```python
from build123d import *

# Parameters (mm, degrees)
FILLET1_R          = 2
FILLET2_R          = 2
REVOLVE3_ANGLE     = 34.5
CUT_EXTRUDE1_START = 17.048322615
CUT_EXTRUDE1_DEPTH = 62.951677385
CUT_EXTRUDE2_REACH = 148.807
SKETCH6_W          = 2.656451676
SKETCH6_H          = 26.566734065
SKETCH6_W_2        = 2.656451675
CUT_EXTRUDE4_DEPTH = 3.1


with BuildPart() as part:
    # Sketch3 → Revolve2 (revolve)
    with BuildSketch(Plane(origin=(0, 0, 0), x_dir=(0, 0, -1), z_dir=(1, 0, 0))):
        with BuildLine():
            Line((0, 0), (36, 0))
            Line((36, 0), (36, 76.3))
            ThreePointArc((36, 76.3), (38.3, 78.6), (36, 80.9))
            Line((36, 80.9), (34.6, 80.9))
            Line((34.6, 80.9), (34.6, 76.3))
            Line((34.6, 76.3), (34.6, 1.4))
            Line((34.6, 1.4), (0, 1.4))
            Line((0, 1.4), (0, 0))
        make_face()
    revolve(axis=Axis((0, 0, 0), (0, 1, 0)))

    # Fillet1
    # the kernel refuses this fillet: 2 mm, written as the material it takes off along each edge
    with BuildSketch(Plane(origin=(0, 80.9, 0), x_dir=(0, 0, -1), z_dir=(1, 0, 0))) as fillet1_piece_1:
        with BuildLine():
            CenterArc((36.6, -1.907878403), FILLET1_R, 107.457603124, 72.542396876)
            Line((34.6, -1.907878403), (34.56, -1.907878403))
            Line((34.56, -1.907878403), (34.56, 0))
            Line((34.56, 0), (34.6, 0.04))
            ThreePointArc((34.6, 0.04), (35.3, 0.04), (35.988, 0.038157568))
            Line((35.988, 0.038157568), (36, 0))
        make_face()
    revolve(axis=Axis((0, 80.9, 0), (0, 1, 0)), mode=Mode.SUBTRACT)

    # Fillet2
    fillet2_edges = [part.edges().sort_by_distance(p)[0] for p in [
        (0, 0, 36),
    ]]
    fillet(fillet2_edges, radius=FILLET2_R)

    # Sketch4 → Revolve3 (revolve)
    with BuildSketch(Plane(origin=(0, 0, 0), x_dir=(0, 0, -1), z_dir=(1, 0, 0))):
        with BuildLine():
            Line((66.418368133, 32.345231294), (37.015359732, 17.048322615))
            Line((37.015359732, 17.048322615), (36, 9))
            Line((36, 9), (36, 19))
            Line((36, 19), (65.403008401, 34.296908679))
            ThreePointArc((65.403008401, 34.296908679), (68.549568046, 37.242877581), (69.710791194, 41.393917351))
            Line((69.710791194, 41.393917351), (69.710791194, 61.739552218))
            ThreePointArc((69.710791194, 61.739552218), (67.034063035, 68.549081537), (60.436853284, 71.71315908))
            Line((60.436853284, 71.71315908), (36, 73.492121597))
            Line((36, 73.492121597), (36, 75.686315107))
            Line((36, 75.686315107), (36.15973366, 75.686315107))
            Line((36.15973366, 75.686315107), (60.596586944, 73.90735259))
            ThreePointArc((60.596586944, 73.90735259), (68.64518284, 70.047177987), (71.910791194, 61.739552218))
            Line((71.910791194, 61.739552218), (71.910791194, 41.393917351))
            ThreePointArc((71.910791194, 41.393917351), (70.43023168, 36.101341644), (66.418368133, 32.345231294))
        make_face()
    revolve(axis=Axis((0, 0, 0), (0, 1, 0)), revolution_arc=REVOLVE3_ANGLE)

    # Cut-Extrude1: read off the stored shape, not the designer's step
    # Cut-Extrude1 outline → Cut-Extrude1 (cut)
    with BuildSketch(Plane(origin=(0, 0, 0), x_dir=(1, 0, 0), z_dir=(0, 1, 0)).offset(CUT_EXTRUDE1_START)):
        with BuildLine():
            Line((-22.108668816, 32.168312739), (-32.047363038, 63.91139403))
            Line((-32.047363038, 63.91139403), (-34.272292741, 63.218445413))
            ThreePointArc((-34.272292741, 63.218445413), (-37.553605301, 61.326084329), (-40.730720635, 59.263566268))
            Line((-40.730720635, 59.263566268), (-22.108668816, 32.168312739))
        make_face()
        with BuildLine():
            Line((0, 38.304663112), (0, 71.910791194))
            ThreePointArc((0, 71.910791194), (-3.848061143, 71.807759438), (-7.685095499, 71.498959414))
            Line((-7.685095499, 71.498959414), (-10.221387179, 70.709037913))
            Line((-10.221387179, 70.709037913), (-0.068922433, 38.283197398))
            Line((-0.068922433, 38.283197398), (0, 38.304663112))
        make_face()
    extrude(amount=CUT_EXTRUDE1_DEPTH, mode=Mode.SUBTRACT)

    # Cut-Extrude2: up to this plane
    cut_extrude2_end = Plane(origin=(-22.697932128, 11.704801269, -66.823250171), z_dir=(0.2973592990807489, 0, 0.9547656504348101))
    # Sketch6 → Cut-Extrude2 (cut, up to the surface)
    with BuildSketch(Plane(origin=(-21.486572607, 0, -68.625717394), x_dir=(-0.9543173737069837, 0, 0.2987948296758254), z_dir=(-0.2987948296758254, 0, -0.9543173737069837)), mode=Mode.PRIVATE) as cut_extrude2_sk1:
        with Locations((-12.701273409, 51.798619412)):
            Rectangle(SKETCH6_W, SKETCH6_H)
    cut_extrude2_tool1 = split(extrude(cut_extrude2_sk1.sketch, amount=-CUT_EXTRUDE2_REACH, mode=Mode.PRIVATE), bisect_by=cut_extrude2_end, keep=Keep.BOTH, mode=Mode.PRIVATE)
    add(cut_extrude2_tool1.solids().sort_by_distance((-9.365527, 51.798619, -72.420792))[0], mode=Mode.SUBTRACT)
    # Sketch6 → Cut-Extrude2 (cut, up to the surface)
    with BuildSketch(Plane(origin=(-21.486572607, 0, -68.625717394), x_dir=(-0.9543173737069837, 0, 0.2987948296758254), z_dir=(-0.2987948296758254, 0, -0.9543173737069837)), mode=Mode.PRIVATE) as cut_extrude2_sk2:
        with Locations((12.815187073, 51.798619412)):
            Rectangle(SKETCH6_W_2, SKETCH6_H)
    cut_extrude2_tool2 = split(extrude(cut_extrude2_sk2.sketch, amount=-CUT_EXTRUDE2_REACH, mode=Mode.PRIVATE), bisect_by=cut_extrude2_end, keep=Keep.BOTH, mode=Mode.PRIVATE)
    add(cut_extrude2_tool2.solids().sort_by_distance((-33.716328, 51.798619, -64.796606))[0], mode=Mode.SUBTRACT)

    # Sketch7 → Cut-Extrude4 (cut)
    with BuildSketch(Plane(origin=(-0.27023011, -1.738396159, -0.863084843), x_dir=(-0.9904458888228052, 0.12351648622229915, 0.06132388560177964), z_dir=(-0.13790192643325755, -0.8871260840574537, -0.4404433785072538))):
        Polygon((30.594390354, 67.226140182), (21.000465395, 34.90437265), (24.682862396, 33.889860102), (33.633833507, 66.37938352), align=None)
        Polygon((5.560376818, 74.302956644), (8.594011842, 73.435621609), (-0.126879919, 40.867445433), (-3.796298497, 41.927940925), align=None)
    extrude(amount=-CUT_EXTRUDE4_DEPTH, mode=Mode.SUBTRACT)


solid = part.part
```
Work out the finished part from the listing and answer in its coordinate system (mm). A direction names the side the tool comes from. Coordinates: 2 decimals unless noted, no trailing zeros. Write each loop counter-clockwise with the first axis right and the second up, starting at its lowest first coordinate (ties: lowest second). Pieces come first, ordered by that corner, then holes.
Q1. A cutting plane is placed at A-A, the plane y = 58. Give the vertices of the cut face in (x, z).
Q2. Each of these flat-tipped pins is pushed along its axis until it touches: pin 1 Ø1 at (x, y) = (20.5, 20) entering from -Z; pin 2 Ø1.3 at (y, z) = (16.5, -37) entering from +X; pin 3 Ø10 at (y, z) = (23, 24) entering from +X. Where does it stop, or does it pass through?
Q3. Which of the six approach directions +Z, -Z, +X, -X, +Y, -Y give full straight-line access (tool end or side, diameter ignored) to faces 1 (the face through (0, 1.4, 0)), 2 (the face through (-20.731, 51.709, -66.557)), 3 (the face through (-13.41, 74.98, -43.83)), 4 (the face through (-14.11, 22.89, -46.13)), 5 (the face through (-21.262, 74.496, -30.936))?
Q4. A cutting plane is placed at B-B, the plane z = 0. Give the vertices of the cut face in (x, y).
Q5. A cutting plane is placed at C-C, the plane y = 11. Give the vertices of the cut face in (x, z).
Q6. Find the intervals of material crossed by line 1 (Y direction, x = -7, z = -56); line 2 (X direction, y = 64, z = -10); line 3 (Z direction, x = -10.5, y = 41.5), in increasing order.
Q7. Determine the mould class of faces 6 (the face through (0, 0, 0)), 7 (the face through (-21.388, 51.424, -68.656)), 8 (the face through (-13.94, 25.06, -45.56)) for opening direction Z: released by +Z, released by -Z, zero draft, split by the parting line, or undercut.
Findings below:
1. outline: circle Ø72 at (0, 0); (-32.17, -64.31) arc R71.91 ccw to (-10.36, -71.16) - (-9.7, -69.03) arc R69.71 cw to (-31.51, -62.18) - close; hole circle Ø69.2 at (0, 0)
2. pin 1: stops at z = -29.93
2. pin 2: stops at x = 0
2. pin 3: stops at x = 30.58
3. face 1: +Y
3. face 2: +X
3. face 3: -Z, -X
3. face 4: -Z, -X, -Y
3. face 5: -X, -Y
4. outline: (-36, 2) arc R2 ccw to (-34, 0) - (34, 0) arc R2 ccw to (36, 2) - (36, 76.3) arc R2.3 ccw to (36, 80.9) arc R2 ccw to (34.6, 78.99) - (34.6, 1.4) - (-34.6, 1.4) - (-34.6, 78.99) arc R2 ccw to (-36, 80.9) arc R2.3 ccw to (-36, 76.3) - close
5. outline: (-20.53, -29.88) arc R36.25 ccw to (0, -36.25) - (0, -36) arc R36 ccw (long way) to (-20.39, -29.67) - close; hole circle Ø69.2 at (0, 0)
6. line 1: y = 27.15 to 29.63, 72 to 74.21
6. line 2: x = -34.58 to -33.12, 33.12 to 34.58
6. line 3: z = -71.14 to -68.92, -34.43 to -32.97, 32.97 to 34.43
7. face 6: zero draft
7. face 7: released by -Z
7. face 8: undercut
